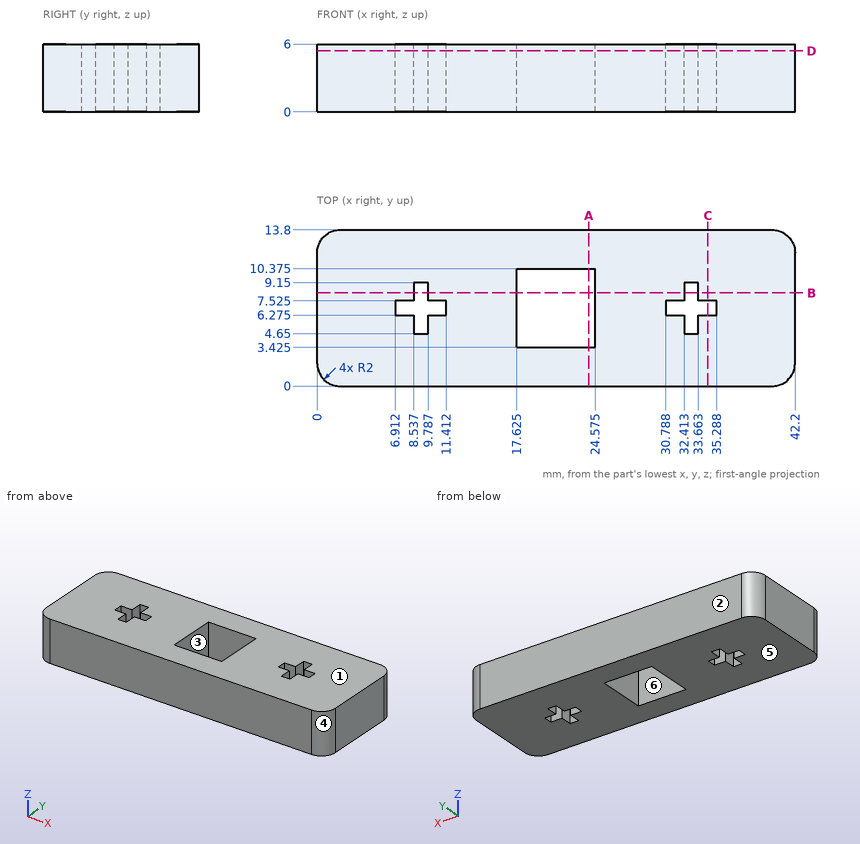
Design review of the part shown in the three views and the two pictorial views. Dimensions are in mm from the part's minimum x, y and z. A direction names the side the tool comes from. Coordinates: 2 decimals unless noted, no trailing zeros. Write each loop counter-clockwise with the first axis right and the second up, starting at its lowest first coordinate (ties: lowest second). Pieces come first, ordered by that corner, then holes. Notation, with made-up numbers: (50.5, 57.25) - (108.5, 57.25) arc R36 ccw to (108.5, 95.25) - close; hole circle Ø5 at (28.25, -0.75). An arc over 180 degrees is marked (long way). Write item = value, one per line.
(1) For line 1 (X direction, y = 8.5, z = 1.6) (3 decimals); line 2 (X direction, y = 7.25, z = 3.7) (3 decimals); line 3 (X direction, y = 10, z = 4.2) (3 decimals), list the stretches that pass through material, from the lowest coordinate up. Write a range as [from, to].
Result sheet:
line_1 = [0, 8.537], [9.787, 17.625], [24.575, 32.413], [33.663, 42.2]
line_2 = [0, 6.912], [11.412, 17.625], [24.575, 30.788], [35.288, 42.2]
line_3 = [0, 17.625], [24.575, 42.2]
(2) Consider section B-B, the plane y = 8.25. Give the boundary of the cut face in (x, z) (3 decimals), then the cut area to 4 significant figures.
Result sheet:
outline = (0, 0) - (8.537, 0) - (8.537, 6) - (0, 6) - close; (9.787, 0) - (17.625, 0) - (17.625, 6) - (9.787, 6) - close; (24.575, 0) - (32.413, 0) - (32.413, 6) - (24.575, 6) - close; (33.663, 0) - (42.2, 0) - (42.2, 6) - (33.663, 6) - close
area = 196.5 mm^2
(3) Consider section C-C, the plane x = 34.5. Give the boundary of the cut face in (y, z) (3 decimals), then the cut area to 3 significant figures.
Result sheet:
outline = (0, 0) - (6.275, 0) - (6.275, 6) - (0, 6) - close; (7.525, 0) - (13.8, 0) - (13.8, 6) - (7.525, 6) - close
area = 75.3 mm^2
(4) Machinability: for the marked faces 5 and 6, which of the approach directions +Z, -Z, +X, -X, +Y, -Y give a long, thin tool a straight path to every point of the face, cutting with its end or side? Answer none if there is none.
Result sheet:
face_5 = -Z, +X, -X, +Y, -Y
face_6 = +Z, -Z
(5) Consider section A-A, the plane x = 24. Give the boundary of the cut face in (y, z) (3 decimals), then the cut area to 3 significant figures.
Result sheet:
outline = (0, 0) - (3.425, 0) - (3.425, 6) - (0, 6) - close; (10.375, 0) - (13.8, 0) - (13.8, 6) - (10.375, 6) - close
area = 41.1 mm^2
(6) For P1, Ø1.8, axis at x = 31.5, z = 2.5, coming from the -Y side, flat-tipped, find the tip position at first contact; note if it passes through.
Result sheet:
P1 = 0
(7) Mouldability with a two-part tool opening along Y and no side actions: class the marked faces 1, 2, 3 and 4 as pulls with the +Y half, pulls with the -Y half, needs draft (parallel to the pull), parting line crosses it, or undercut.
Result sheet:
face_1 = needs draft
face_2 = pulls with the +Y half
face_3 = undercut
face_4 = pulls with the -Y half
(8) Consider section D-D, the plane z = 5.4. State how many separate pieces and enclosed holes the cut face has, then the cut area to 3 significant figures.
Result sheet:
separate_pieces = 1
enclosed_holes = 3
area = 511 mm^2
